from build123d import *

# Parameters (mm, degrees)
F1_W     = 90
F1_H     = 75
F1_R     = 3.15
F2_DEPTH = 4
F3_W     = 19.1
F3_H     = 19.1
F4_W     = 19
F4_H     = 19
F4_W_2   = 19.1
F4_H_2   = 19.1
F5_DEPTH = 0.1
F6_W     = 18.8
F6_H     = 18.8
F7_DEPTH = 0.1


with BuildPart() as f2:
    # F1 (on face) → F2 (new body)
    with BuildSketch(Plane.XY):
        with Locations((-1.603169, 10.190485)):
            Rectangle(F1_W, F1_H)
        with Locations((-37.603169, -19.059515)):
            Circle(F1_R, mode=Mode.SUBTRACT)
        with Locations((34.396831, -19.059515)):
            Circle(F1_R, mode=Mode.SUBTRACT)
        with Locations((-37.603169, 39.440485)):
            Circle(F1_R, mode=Mode.SUBTRACT)
        with Locations((34.396831, 39.440485)):
            Circle(F1_R, mode=Mode.SUBTRACT)
    extrude(amount=F2_DEPTH)

    # F3 (on face) + F4 (on face) → F5 (cut)
    with BuildSketch(Plane.XY.offset(4)):
        with Locations((-1.493169, 10.050485)):
            Rectangle(F3_W, F3_H)
    with BuildSketch(Plane.XY.offset(4)):
        with Locations((-1.496693, 10.04078)):
            Rectangle(F4_W, F4_H)
        with Locations((-1.493169, 10.050485)):
            Rectangle(F4_W_2, F4_H_2)
        with Locations((-1.496693, 10.04078)):
            Rectangle(F4_W, F4_H, mode=Mode.SUBTRACT)
    extrude(amount=-F5_DEPTH, mode=Mode.SUBTRACT)

    # F6 (on face) → F7 (join)
    with BuildSketch(Plane.XY.offset(3.9)):
        with Locations((-1.504565, 10.029633)):
            Rectangle(F6_W, F6_H)
    extrude(amount=F7_DEPTH)


solid = f2.part
Read the model definition and answer for the solid it produces. Units are mm, in the model's axes. Round coordinates to 2 decimals unless told otherwise and drop trailing zeros. Write each loop counter-clockwise with the first axis right and the second up, starting at its lowest first coordinate (ties: lowest second). Pieces come first, ordered by that corner, then holes.
Q1. Find section C-C on z = 1.95. Determine the outline of the cut face in (x, y).
Values:
outline: (-46.6, -27.31) - (43.4, -27.31) - (43.4, 47.69) - (-46.6, 47.69) - close; hole circle Ø6.3 at (-37.6, -19.06); hole circle Ø6.3 at (-37.6, 39.44); hole circle Ø6.3 at (34.4, -19.06); hole circle Ø6.3 at (34.4, 39.44)
Q2. Find section A-A on x = 36. Determine the outline of the cut face in (y, z), and give its area (3 significant figures).
Values:
outline: (-27.31, 0) - (-21.77, 0) - (-21.77, 4) - (-27.31, 4) - close; (-16.35, 0) - (36.73, 0) - (36.73, 4) - (-16.35, 4) - close; (42.15, 0) - (47.69, 0) - (47.69, 4) - (42.15, 4) - close
area: 257 mm2
Q3. A flat-ended cylindrical pin translates along its axis: P1, Ø4, axis at x = 34.4, y = 39.44, coming from the -Z side. Find the tip coordinate at first contact, or state that the pin passes through.
Values:
P1: passes through
Q4. The mould has two halves that part along Y. Classify faces 1 (the face through (43.397, 10, 2)), 2 (the face through (-2, 47.69, 2)), 3 (the face through (-36.15, -21.854, 1.972)), 4 (the face through (35.85, -21.854, 1.972)): released by +Y, released by -Y, zero draft, split by the parting line, or undercut.
Values:
face 1: zero draft
face 2: released by +Y
face 3: undercut
face 4: undercut
Q5. Straight lines are drawn through the part: line 1 (X direction, y = -19, z = 0.35); line 2 (X direction, y = 40, z = 1.2); line 3 (Y direction, x = -39, z = 2.3). For each, find the intervals that lie inside material, in ascending order.
Values:
line 1: x = -46.6 to -40.75, -34.45 to 31.25, 37.55 to 43.4
line 2: x = -46.6 to -40.7, -34.5 to 31.3, 37.5 to 43.4
line 3: y = -27.31 to -21.88, -16.24 to 36.62, 42.26 to 47.69
Q6. Find section B-B on y = -20. Determine the outline of the cut face in (x, z), and give its area (3 significant figures).
Values:
outline: (-46.6, 0) - (-40.61, 0) - (-40.61, 4) - (-46.6, 4) - close; (-34.6, 0) - (31.39, 0) - (31.39, 4) - (-34.6, 4) - close; (37.4, 0) - (43.4, 0) - (43.4, 4) - (37.4, 4) - close
area: 312 mm2
